Check sheet for the modelled part. Datum: model origin and axes. Units: mm. Coordinates: 2 decimals unless noted, no trailing zeros. Loops run counter-clockwise (first coordinate to the right, second up) from the corner with the lowest first, then second, coordinate; pieces in that order, holes last.
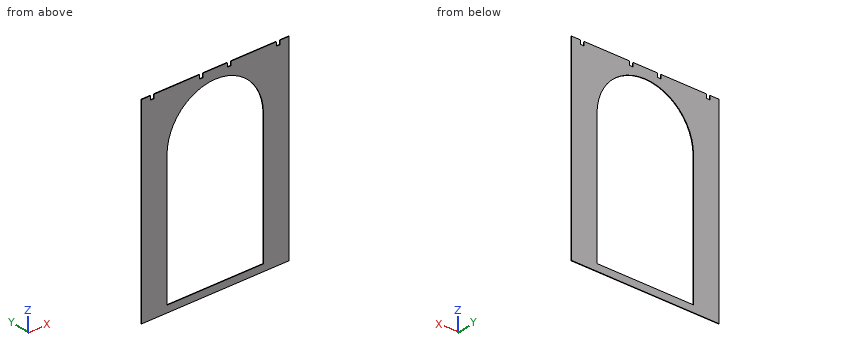
```python
from build123d import *

# Parameters (mm, degrees)
F1_DEPTH = 3


with BuildPart() as f1:
    # F0 (on Front) → F1 (new body)
    with BuildSketch(Plane.XZ):
        Polygon((0, 1000), (0, 0), (750, 0), (750, 1000), (704, 1000), (704, 980), (685, 980), (685, 1000), (455, 1000), (455, 980), (436, 980), (436, 1000), (314, 1000), (314, 980), (295, 980), (295, 1000), (65, 1000), (65, 980), (46, 980), (46, 1000), align=None)
        with BuildLine():
            Line((620, 35), (130, 35))
            Line((130, 35), (130, 705))
            ThreePointArc((130, 705), (375, 950), (620, 705))
            Line((620, 705), (620, 35))
        make_face(mode=Mode.SUBTRACT)
    extrude(amount=F1_DEPTH)


solid = f1.part
```
1) Section check B-B on z = 377. Enter the section's corners in (x, y), plus the area to 3 significant figures.
Answer sheet:
outline: (0, -3) - (130, -3) - (130, 0) - (0, 0) - close; (620, -3) - (750, -3) - (750, 0) - (620, 0) - close
area: 780 mm2
2) Section check C-C on y = -2.2. Enter the section's corners in (x, z), plus the area to 3 significant figures.
Answer sheet:
outline: (0, 0) - (750, 0) - (750, 1000) - (704, 1000) - (704, 980) - (685, 980) - (685, 1000) - (455, 1000) - (455, 980) - (436, 980) - (436, 1000) - (314, 1000) - (314, 980) - (295, 980) - (295, 1000) - (65, 1000) - (65, 980) - (46, 980) - (46, 1000) - (0, 1000) - close; hole (130, 35) - (620, 35) - (620, 705) arc R245 ccw to (130, 705) - close
area: 326,000 mm2
3) Section check A-A on x = 375. Enter the section's corners in (y, z), plus the area to 3 significant figures.
Answer sheet:
outline: (-3, 0) - (0, 0) - (0, 35) - (-3, 35) - close; (-3, 950) - (0, 950) - (0, 1000) - (-3, 1000) - close
area: 255 mm2
4) Scan lines: line 1 (X direction, y = -2.25, z = 281.5); line 2 (X direction, y = -1.1, z = 809.5); line 3 (Z direction, x = 180, y = -0.85). Record each from-to range of solid material in increasing order.
Answer sheet:
line 1: x = 0 to 130, 620 to 750
line 2: x = 0 to 153.4, 596.6 to 750
line 3: z = 0 to 35, 853.32 to 1000
5) Depth check by flat-ended pin: pin 1 (1.5 mm diameter, centred on x = 300.5, y = -2, fed in from +Z). Enter the tip coordinate at first touch or a pass-through.
Answer sheet:
pin 1: stops at z = 980
